```python
from build123d import *

# Parameters (mm, degrees)
SKETCH1_R           = 25
BOSS_EXTRUDE1_DEPTH = 70
SKETCH3_R           = 25
BOSS_EXTRUDE2_DEPTH = 75
CHAMFER1_SIZE       = 10


with BuildPart() as part:
    # Sketch1 → Boss-Extrude1 (new body)
    with BuildSketch(Plane(origin=(0, 0, 0), x_dir=(1, 0, 0), z_dir=(0, 1, 0))):
        Polygon((70, 0), (-70, 0), (-70, -20), (-50, -20), (-50, -70), (50, -70), (50, -20), (70, -20), align=None)
        with Locations((0, -35)):
            Circle(SKETCH1_R, mode=Mode.SUBTRACT)
    extrude(amount=BOSS_EXTRUDE1_DEPTH)

    # Sketch3 → Boss-Extrude2 (add, symmetric)
    with BuildSketch(Plane(origin=(0, 35, 0), x_dir=(1, 0, 0), z_dir=(0, 1, 0))):
        with Locations((0, -35)):
            Circle(SKETCH3_R)
    extrude(amount=BOSS_EXTRUDE2_DEPTH, both=True)

    # Sketch4 → Revolve1 (revolve)
    with BuildSketch(Plane.XY.offset(35)):
        Polygon((-9.564011188, 110), (0, 110), (0, 133.766089862), (-6.754803398, 133.766089862), (-6.754803398, 123.383600129), (-9.564011188, 123.383600129), (-9.564011188, 118.357377814), (-8.389537285, 118.357377814), (-8.389537285, 114.668590284), (-9.564011188, 114.668590284), align=None)
        Polygon((0, -40), (-9.564011188, -40), (-9.564011188, -50.700633695), (-4.891534663, -50.700633695), (-4.891534663, -52.417938892), (0, -52.417938892), align=None)
    revolve(axis=Axis((0, -40, 35), (0, -1, 0)))

    # Chamfer1
    chamfer1_edges = [part.edges().sort_by_distance(p)[0] for p in [
        (50, 35, 70),
        (-50, 35, 70),
    ]]
    chamfer(chamfer1_edges, length=CHAMFER1_SIZE)


solid = part.part
```
Design review of the part built by this model. Coordinates are the model's own, in mm. A direction names the side the tool comes from. Round coordinates to 2 decimals unless told otherwise and drop trailing zeros. Write each loop counter-clockwise with the first axis right and the second up, starting at its lowest first coordinate (ties: lowest second). Pieces come first, ordered by that corner, then holes. Notation, with made-up numbers: (62.5, 77) -> (116.5, 77) arc R34 ccw to (116.5, 113) -> close; hole circle Ø5 at (26, -33.5). An arc over 180 degrees is marked (long way). Write item = value, one per line. Start each with the question number.
1) Take a section at A-A, the plane y = 49. State the section outline as (x, z) points, plus the area to 3 significant figures.
2) Take a section at D-D, the plane y = -29.5. State the section outline as (x, z) points.
3) Mouldability with a two-part tool opening along Y and no side actions: class faces 6 (the face through (60, 35, 20)), 7 (the face through (-3, 118.357, 43)), 8 (the face through (0, 133.766, 35)) as +Y half, -Y half, draft (parallel to the pull), parting line (faces both ways), or undercut.
4) Tool access review of faces 1 (the face through (-4, -50.701, 39)), 2 (the face through (0, 110, 46)), 3 (the face through (-50, 35, 40)), 4 (the face through (3, 114.669, 43)), 5 (the face through (50, 35, 40)): name each direction out of +Z, -Z, +X, -X, +Y, -Y from which nothing blocks a thin tool from reaching the whole face with its end or side.
5) Take a section at B-B, the plane x = 28. State the section outline as (y, z) points, plus the area to 3 significant figures.
6) Wall thickness on probe 1 along Y at (x, z) = (-39, 17); probe 2 along Y at (x, z) = (4, 53.5); probe 3 along X at (y, z) = (95, 49.5): over which ranges is each line inside the solid? List them lowest first. Write a range as from..to.
7) Clearance check with flat-ended pins moving along their axes: pin 1 (5 mm diameter, centred on x = 45, y = 13, fed in from +Z); pin 2 (10 mm diameter, centred on x = 36, z = 26.5, fed in from -Y); pin 3 (10 mm diameter, centred on x = 57, y = 37.5, fed in from +Z). State where each tip first meets the part, or that it passes through.
8) Take a section at C-C, the plane z = 17.5. State the section outline as (x, y) points, plus the area to 3 significant figures.
Results list:
q1.outline = (-70, 0) -> (70, 0) -> (70, 20) -> (50, 20) -> (50, 60) -> (40, 70) -> (-40, 70) -> (-50, 60) -> (-50, 20) -> (-70, 20) -> close
q1.area = 7,700 mm²
q2.outline = circle Ø50 at (0, 35)
q3.face_6 = draft
q3.face_7 = undercut
q3.face_8 = +Y half
q4.face_1 = -Y
q4.face_2 = +Y
q4.face_3 = +Z, -X, +Y, -Y
q4.face_4 = none
q4.face_5 = +Z, +X, +Y, -Y
q5.outline = (0, 0) -> (70, 0) -> (70, 70) -> (0, 70) -> close
q5.area = 4,900 mm²
q6.probe_1 = 0..70
q6.probe_2 = -40..110
q6.probe_3 = -20.37..20.37
q7.pin_1 = 67.5
q7.pin_2 = 0
q7.pin_3 = 20
q8.outline = (-70, 0) -> (-17.85, 0) -> (-17.85, -40) -> (17.85, -40) -> (17.85, 0) -> (70, 0) -> (70, 70) -> (17.85, 70) -> (17.85, 110) -> (-17.85, 110) -> (-17.85, 70) -> (-70, 70) -> close
q8.area = 12,700 mm²
